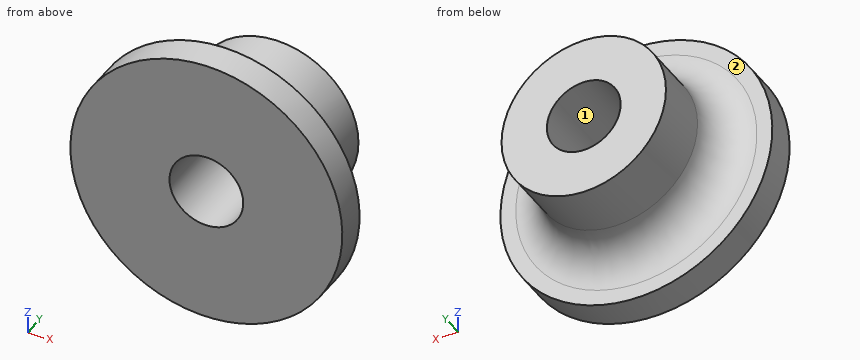
from build123d import *

# Parameters (mm, degrees)
F0_W   = 15.167773
F0_H   = 25.785211
F0_H_2 = 21.740476
F0_W_2 = 46.13531
F2_R   = 18.396307


with BuildPart() as f1:
    # F0 (on Right) → F1 (revolve)
    with BuildSketch(Plane.YZ):
        with Locations((-53.719196, 52.328815)):
            Rectangle(F0_W, F0_H)
        with Locations((-53.719196, 28.565972)):
            Rectangle(F0_W, F0_H_2)
        with Locations((-23.067655, 28.565972)):
            Rectangle(F0_W_2, F0_H_2)
    revolve(axis=Axis((0, -30.651541, 0), (0, -1, 0)))

    # F2
    f2_edges = [f1.edges().sort_by_distance(p)[0] for p in [
        (0, -46.13531, -39.43621),
    ]]
    fillet(f2_edges, radius=F2_R)


solid = f1.part
CAD build for the part. Positions are in the model's coordinates, mm. Face numbers are marked on the shaded views. A direction names the side the tool comes from. Coordinates: 2 decimals unless noted, no trailing zeros. Write each loop counter-clockwise with the first axis right and the second up, starting at its lowest first coordinate (ties: lowest second). Pieces come first, ordered by that corner, then holes. Notation, with made-up numbers: (21.5, -24.75) - (64.5, -24.75) arc R19 ccw to (64.5, -11.75) - close; hole circle Ø10 at (-31, -12). An arc over 180 degrees is marked (long way). Use a Markdown table: item, result. Add a question column.
Item 1: Drill centre lines: L1, parallel to Z at x = 0, y = -19.5; L2, parallel to X at y = -48, z = 0. Where is each one in solid material? Low to high. Write a range as from..to.
Item 2: Band-saw the part on A-A, the plane x = 0. Give the cut face in (y, z).
Item 3: Band-saw the part on C-C, the plane y = -24.5. Give the cut face in (x, z), and give its area (3 significant figures).
Item 4: Flat gauge pins, fed straight in: pin 1 (8 mm diameter, centred on y = -49, z = 38, fed in from +X); pin 2 (3 mm diameter, centred on y = -45, z = 48.5, fed in from +X); pin 3 (6 mm diameter, centred on x = -50.5, y = -48, fed in from +Z). Where does each tip first touch, or does it go through?
Item 5: 3-axis set-ups, long thin cutter, end or side, ignore diameter. For the marked faces 1 and 2: which of +Z, -Z, +X, -X, +Y, -Y reach the whole face in a straight line?
Item 6: Band-saw the part on B-B, the plane z = 0. Give the cut face in (x, y).
Item 7: Band-saw the part on D-D, the plane y = -48.5. Give the cut face in (x, z), and give its area (3 significant figures).
Numbers:
| question | item | result |
|---|---|---|
| 1 | L1 | -39.44..-17.7, 17.7..39.44 |
| 1 | L2 | -65.22..-17.7, 17.7..65.22 |
| 2 | outline | (-61.3, -65.22) - (-46.14, -65.22) - (-46.14, -57.83) arc R18.4 cw to (-27.74, -39.44) - (0, -39.44) - (0, -17.7) - (-61.3, -17.7) - close; (-61.3, 17.7) - (0, 17.7) - (0, 39.44) - (-27.74, 39.44) arc R18.4 cw to (-46.14, 57.83) - (-46.14, 65.22) - (-61.3, 65.22) - close |
| 3 | outline | circle Ø78.87 at (0, 0); hole circle Ø35.39 at (0, 0) |
| 3 | area | 3,900 mm2 |
| 4 | pin 1 | x = 55.66 |
| 4 | pin 2 | x = 44.67 |
| 4 | pin 3 | z = 44.69 |
| 5 | face 1 | +Y, -Y |
| 5 | face 2 | +Y |
| 6 | outline | (-65.22, -61.3) - (-17.7, -61.3) - (-17.7, 0) - (-39.44, 0) - (-39.44, -27.74) arc R18.4 cw to (-57.83, -46.14) - (-65.22, -46.14) - close; (17.7, -61.3) - (65.22, -61.3) - (65.22, -46.14) - (57.83, -46.14) arc R18.4 cw to (39.44, -27.74) - (39.44, 0) - (17.7, 0) - close |
| 7 | outline | circle Ø130.44 at (0, 0); hole circle Ø35.39 at (0, 0) |
| 7 | area | 12,400 mm2 |
